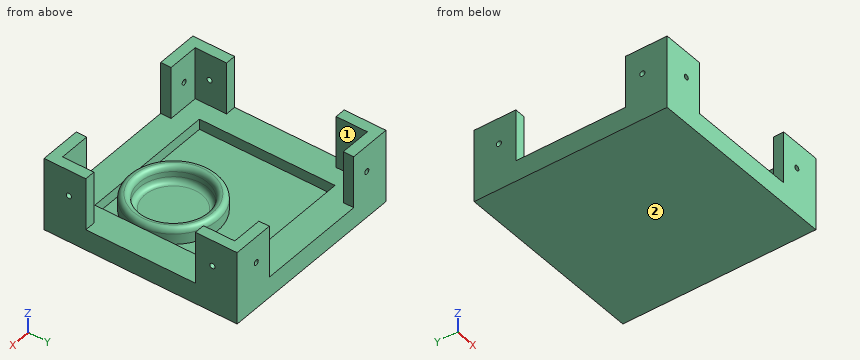
Autodesk Inventor part; units mm, degrees
ref_plane "YZ Plane" through (0, 0, 0) normal (1, 0, 0) x (0, 1, 0)
ref_plane "XZ Plane" through (0, 0, 0) normal (0, 1, 0) x (-1, 0, 0)
ref_plane "XY Plane" through (0, 0, 0) normal (0, 0, 1) x (1, 0, 0)
sketch "Sketch2" plane through (0, 0, 0) normal (0, 0, 1) x (1, 0, 0)
  line L0 (-37, 37) -> (37, 37)
  line L1 (37, 37) -> (37, -37)
  line L2 (37, -37) -> (-37, -37)
  line L3 (-37, -37) -> (-37, 37)
  point P0 (0, 0)
  point P1 (0, 37)
  point P2 (37, 0)
  dimension "d0" = 74
  dimension "d1" = 74
extrude "Extrusion1" add sketch "Sketch2" along normal blind 8
sketch "Sketch3" plane through (0, 0, 8) normal (0, 0, 1) x (1, 0, 0)
  line L0 (-37, 37) -> (-21, 37)
  line L1 (-21, 37) -> (-21, 33)
  line L2 (-21, 33) -> (-37, 33)
  line L3 (-37, 33) -> (-37, 37)
  line L4 (-37, 37) -> (-37, -37) construction
  line L5 (37, 37) -> (-37, 37) construction
  line L6 (-37, 33) -> (-33, 33)
  line L7 (-33, 33) -> (-33, 21)
  line L8 (-33, 21) -> (-37, 21)
  line L9 (-37, 21) -> (-37, 33)
  line L10 (21, 33) -> (21, 37)
  line L11 (21, 37) -> (33, 37)
  line L12 (33, 37) -> (33, 33)
  line L13 (33, 33) -> (21, 33)
  line L14 (33, 21) -> (33, 37)
  line L15 (37, 21) -> (33, 21)
  line L16 (37, 37) -> (37, 21)
  line L17 (33, 37) -> (37, 37)
  line L18 (33, -21) -> (37, -21)
  line L19 (37, -21) -> (37, -33)
  line L20 (37, -33) -> (33, -33)
  line L21 (33, -33) -> (33, -21)
  line L22 (21, -33) -> (37, -33)
  line L23 (21, -37) -> (21, -33)
  line L24 (37, -37) -> (21, -37)
  line L25 (37, -33) -> (37, -37)
  line L26 (-21, -33) -> (-21, -37)
  line L27 (-21, -37) -> (-33, -37)
  line L28 (-33, -37) -> (-33, -33)
  line L29 (-33, -33) -> (-21, -33)
  line L30 (-33, -21) -> (-33, -37)
  line L31 (-37, -21) -> (-33, -21)
  line L32 (-37, -37) -> (-37, -21)
  line L33 (-33, -37) -> (-37, -37)
  point P0 (0, 0)
  point P1 (0, 0)
  point P2 (0, 0)
  point P3 (0, 0)
  dimension "d4" = 0
  dimension "d5" = 16
  dimension "d6" = 4
  dimension "d8" = 4
  dimension "d9" = 12
  dimension "d12" = 360
extrude "Extrusion2" add sketch "Sketch3" along normal blind 20
sketch "Sketch4" plane through (-37, -37, 0) normal (-1, 0, 0) x (0, 0, 1)
  circle A0 centre (18, 64.5) radius 1
  line L0 (28, 74) -> (28, 58)
  line L1 (8, 58) -> (8, 16)
  line L2 (0, 37) -> (20, 37) construction
  line L3 (0, 37) -> (20, 37) construction
  circle A1 centre (18, 9.5) radius 1
  line L4 (0, 74) -> (28, 74)
  dimension "d16" = 2
  dimension "d18" = 10
  dimension "d19" = 20
  dimension "d20" = 0
  dimension "d26" = 9.5
extrude "Extrusion3" cut sketch "Sketch4" against normal up to surface (4 mm away)
pattern_circular "Circular Pattern1" count 4 over 360 about axis through (0, 0, -10) along (0, 0, 1) of "Extrusion3"
sketch "Sketch5" plane through (0, 0, 8) normal (0, 0, 1) x (1, 0, 0)
  line L0 (-26, -26) -> (26, -26)
  line L1 (26, -26) -> (26, 26)
  line L2 (26, 26) -> (-26, 26)
  line L3 (-26, 26) -> (-26, -26)
  line L4 (-21, -37) -> (21, -37)
  line L5 (-37, 21) -> (-37, -21)
  point P0 (0, 0)
  point P1 (-26, 0)
  point P2 (0, 26)
  dimension "d27" = 11
  dimension "d28" = 11
extrude "Extrusion4" cut sketch "Sketch5" against normal blind 4
sketch "Sketch8" plane through (0, 0, 4) normal (0, 0, 1) x (1, 0, 0)
  circle A0 centre (9, -9) radius 17
  line L0 (26, -26) -> (-26, -26)
  line L1 (26, 26) -> (26, -26)
  circle A1 centre (9, -9) radius 13
  point P0 (0, 0)
  dimension "d49" = 34
  dimension "d50" = 26
extrude "Extrusion7" add sketch "Sketch8" along normal blind 6 contours A0
fillet "Fillet1" radius 2 2 edges at (-4, -9, 10) (-8, -9, 10)
fillet "Fillet2" radius 2 1 edges at (-4, -9, 4)
equation "\"d1\" = d0"
equation "\"d8\" = d6"
equation "\"d9\" = d5 - d6"
properties part number "Bottom"
For this review, take the finished solid that the model builds, in its own axes (mm). Face numbers are marked on the shaded views. A direction names the side the tool comes from. Round coordinates to 2 decimals unless told otherwise and drop trailing zeros. Loops run counter-clockwise (first coordinate to the right, second up) from the corner with the lowest first, then second, coordinate; pieces in that order, holes last. Notation, with made-up numbers: (28.5, -20.75) - (40.5, -20.75) arc R10 cw to (40.5, -1.75) - close; hole circle Ø1 at (-1, 81). An arc over 180 degrees is marked (long way). One line per item, written item: value. Start each with the question number.
Item 1: Take a section at A-A (x = -27.5). Give the boundary of the cut face in (y, z), plus the area to 3 significant figures.
Item 2: Take a section at D-D (x = -13). Give the boundary of the cut face in (y, z).
Item 3: Take a section at C-C (z = 26). Give the boundary of the cut face in (x, y), plus the area to 3 significant figures.
Item 4: For L1, parallel to Y at x = -34.05, z = 18; L2, parallel to X at y = 33.5, z = 26; L3, parallel to Z at x = 34.3, y = 27.5, list the stretches that pass through material, from the lowest coordinate up.
Item 5: For the marked faces 1 and 2, list the 3-axis set-ups (+Z, -Z, +X, -X, +Y, -Y) from which the entire face can be reached by the end or side of a thin tool; tool diameter is ignored.
Item 6: Clearance check with flat-ended pins moving along their axes: pin 1 Ø15 at (x, y) = (11, -2.5) entering from +Z; pin 2 Ø5 at (x, y) = (-5, 12) entering from -Z; pin 3 Ø12 at (x, y) = (-16.5, 7.5) entering from +Z; pin 4 Ø5 at (x, y) = (18, -19.5) entering from +Z. State where each tip first meets the part, or that it passes through.
Answer below:
1. outline: (-37, 0) - (37, 0) - (37, 17) - (33, 17) - (33, 8) - (-33, 8) - (-33, 17) - (-37, 17) - close; (-37, 19) - (-33, 19) - (-33, 28) - (-37, 28) - close; (33, 19) - (37, 19) - (37, 28) - (33, 28) - close
1. area: 736 mm2
2. outline: (-37, 0) - (37, 0) - (37, 8) - (26, 8) - (26, 4) - (-26, 4) - (-26, 8) - (-37, 8) - close
3. outline: (-37, -37) - (-21, -37) - (-21, -33) - (-33, -33) - (-33, -21) - (-37, -21) - close; (-37, 21) - (-33, 21) - (-33, 33) - (-21, 33) - (-21, 37) - (-37, 37) - close; (21, -37) - (37, -37) - (37, -21) - (33, -21) - (33, -33) - (21, -33) - close; (21, 33) - (33, 33) - (33, 21) - (37, 21) - (37, 37) - (21, 37) - close
3. area: 448 mm2
4. L1: y = -37 to -28.5, -26.5 to -21, 21 to 26.5, 28.5 to 37
4. L2: x = -37 to -21, 21 to 37
4. L3: z = 0 to 17, 19 to 28
5. face 1: +Z
5. face 2: -Z, +X, -X, +Y, -Y
6. pin 1: stops at z = 9.87
6. pin 2: stops at z = 0
6. pin 3: stops at z = 4
6. pin 4: stops at z = 10
